from build123d import *

# Parameters (mm, degrees)
BOSS_EXTRUDE1_DEPTH = 104.85
CUT_EXTRUDE1_REACH  = 178.992
CUT_EXTRUDE2_REACH  = 178.992
SKETCH3_R           = 2.665000000000001
BOSS_EXTRUDE2_DEPTH = 104.85
CUT_EXTRUDE3_REACH  = 178.992
SKETCH6_W           = 66.67499999999998
SKETCH6_H           = 36.500000000000014
CUT_EXTRUDE4_DEPTH  = 3.5
CUT_EXTRUDE5_DEPTH  = 94.850000094
SKETCH9_R           = 2.7500000000000084
SKETCH9_R_2         = 2.750000000000008
CUT_EXTRUDE6_DEPTH  = 5
CUT_EXTRUDE7_DEPTH  = 99.85
BOSS_EXTRUDE3_DEPTH = 40
SKETCH12_R          = 19.05
BOSS_EXTRUDE4_DEPTH = 76.2
CHAMFER1_SIZE       = 13.43611593
CHAMFER1_SIZE_2     = 76.2
CUT_EXTRUDE8_REACH  = 166.091
SKETCH13_R          = 8.750000000000004
CUT_EXTRUDE9_REACH  = 166.091
SKETCH14_R          = 1.7500000000000038
SKETCH14_R_2        = 1.7500000000000067
SKETCH14_R_3        = 1.7499999999999987


# Read off the part's stored shape, not the designer's step: Shell1
with BuildPart() as part:
    # Sketch1 → Boss-Extrude1 (new body)
    with BuildSketch(Plane.XY):
        with BuildLine():
            Line((-34.925, 0), (-34.92499999999999, -63.5))
            Line((-34.92499999999999, -63.5), (-34.92499999999998, -103.175))
            Line((-34.92499999999998, -103.175), (98.425, -103.175))
            Line((98.425, -103.175), (98.42499999999998, -64.83388883768319))
            Line((98.42499999999998, -64.83388883768319), (98.425, 0))
            ThreePointArc((98.425, 0), (31.750000000000004, 66.675), (-34.925, 0))
        make_face()
    extrude(amount=BOSS_EXTRUDE1_DEPTH)

    # Sketch2 → Cut-Extrude1 (cut, up to next)
    with BuildSketch(Plane.XY.offset(104.85), mode=Mode.PRIVATE) as cut_extrude1_sk1:
        with BuildLine():
            Line((31.75, -66.675), (31.75, -103.175))
            Line((31.75, -103.175), (98.425, -103.175))
            Line((98.425, -103.175), (98.425, 0))
            ThreePointArc((98.425, 0), (78.89634463561305, -47.14634463561305), (31.75, -66.675))
        make_face()
    cut_extrude1_tool1 = extrude(cut_extrude1_sk1.sketch, amount=-CUT_EXTRUDE1_REACH, mode=Mode.PRIVATE) & part.part
    add(cut_extrude1_tool1.solids().sort_by_distance((70.281775, -75.59134, 104.85))[0], mode=Mode.SUBTRACT)

    # Sketch3 → Cut-Extrude2 (cut, up to next)
    with BuildSketch(Plane(origin=(0, 0, 0), x_dir=(-1, 0, 0), z_dir=(0, 0, -1)), mode=Mode.PRIVATE) as cut_extrude2_sk1:
        with Locations((-21.75, -93.17500000000001)):
            Circle(SKETCH3_R)
    cut_extrude2_tool1 = extrude(cut_extrude2_sk1.sketch, amount=-CUT_EXTRUDE2_REACH, mode=Mode.PRIVATE) & part.part
    # Sketch3 → Cut-Extrude2 (cut, up to next)
    with BuildSketch(Plane(origin=(0, 0, 0), x_dir=(-1, 0, 0), z_dir=(0, 0, -1)), mode=Mode.PRIVATE) as cut_extrude2_sk2:
        with Locations(Location((-21.75, -73.17499999999998, 0), (0, 0, 180))):
            Circle(SKETCH3_R)
    cut_extrude2_tool2 = extrude(cut_extrude2_sk2.sketch, amount=-CUT_EXTRUDE2_REACH, mode=Mode.PRIVATE) & part.part
    # Sketch3 → Cut-Extrude2 (cut, up to next)
    with BuildSketch(Plane(origin=(0, 0, 0), x_dir=(-1, 0, 0), z_dir=(0, 0, -1)), mode=Mode.PRIVATE) as cut_extrude2_sk3:
        with Locations(Location((24.924999999999997, -93.17500000000001, 0), (0, 0, 180))):
            Circle(SKETCH3_R)
    cut_extrude2_tool3 = extrude(cut_extrude2_sk3.sketch, amount=-CUT_EXTRUDE2_REACH, mode=Mode.PRIVATE) & part.part
    # Sketch3 → Cut-Extrude2 (cut, up to next)
    with BuildSketch(Plane(origin=(0, 0, 0), x_dir=(-1, 0, 0), z_dir=(0, 0, -1)), mode=Mode.PRIVATE) as cut_extrude2_sk4:
        with Locations((24.924999999999997, -73.17499999999998)):
            Circle(SKETCH3_R)
    cut_extrude2_tool4 = extrude(cut_extrude2_sk4.sketch, amount=-CUT_EXTRUDE2_REACH, mode=Mode.PRIVATE) & part.part
    add(cut_extrude2_tool1.solids().sort_by_distance((21.75, -93.175, 0))[0], mode=Mode.SUBTRACT)
    add(cut_extrude2_tool2.solids().sort_by_distance((21.75, -73.175, 0))[0], mode=Mode.SUBTRACT)
    add(cut_extrude2_tool3.solids().sort_by_distance((-24.925, -93.175, 0))[0], mode=Mode.SUBTRACT)
    add(cut_extrude2_tool4.solids().sort_by_distance((-24.925, -73.175, 0))[0], mode=Mode.SUBTRACT)

    # Sketch5 → Boss-Extrude2 (add)
    with BuildSketch(Plane(origin=(0, 0, 0), x_dir=(-1, 0, 0), z_dir=(0, 0, -1))):
        with BuildLine():
            Line((-31.75, -66.675), (-98.425, -66.675))
            Line((-98.425, -66.675), (-98.425, -4.6559e-13))
            ThreePointArc((-98.425, -4.6559e-13), (-78.89634463561288, -47.146344635613225), (-31.75, -66.675))
        make_face()
    extrude(amount=-BOSS_EXTRUDE2_DEPTH)

    # Sketch6 → Cut-Extrude3 (cut, up to next)
    with BuildSketch(Plane(origin=(0, 0, 0), x_dir=(-1, 0, 0), z_dir=(0, 0, -1)), mode=Mode.PRIVATE) as cut_extrude3_sk1:
        with Locations((1.5874999999999897, -84.92500000000001)):
            Rectangle(SKETCH6_W, SKETCH6_H)
    cut_extrude3_tool1 = extrude(cut_extrude3_sk1.sketch, amount=-CUT_EXTRUDE3_REACH, mode=Mode.PRIVATE) & part.part
    add(cut_extrude3_tool1.solids().sort_by_distance((-1.5875, -84.925, 0))[0], mode=Mode.SUBTRACT)

    # Sketch7 → Cut-Extrude4 (cut)
    with BuildSketch(Plane.XZ.offset(66.675)):
        Polygon((98.425, 0), (98.425, 104.85), (-34.92499999999999, 104.85), (-34.92499999999998, 0), align=None)
    extrude(amount=-CUT_EXTRUDE4_DEPTH, mode=Mode.SUBTRACT)

    # Sketch8 → Cut-Extrude5 (cut)
    with BuildSketch(Plane(origin=(0, 0, 4.999999905999999), x_dir=(-1, 0, 0), z_dir=(0, 0, -1))):
        with BuildLine():
            Line((-98.425, -20.224984548819855), (-98.425, -60.17499999999999))
            Line((-98.425, -60.17499999999999), (-66.87228637204589, -60.17499999999999))
            ThreePointArc((-66.87228637204589, -60.17500000000001), (-86.42790057980886, -43.18486787272293), (-98.42499999999998, -20.224984548819855))
        make_face()
    extrude(amount=-CUT_EXTRUDE5_DEPTH, mode=Mode.SUBTRACT)

    # Sketch9 → Cut-Extrude6 (cut)
    with BuildSketch(Plane(origin=(0, -60.17499999999999, 0), x_dir=(1, 0, 0), z_dir=(0, 1, 0))):
        with Locations(Location((89.99999999999999, -89.85, 0), (0, 0, 270))):
            Circle(SKETCH9_R)
        with Locations(Location((89.99999999999999, -14.999999906000001, 0), (0, 0, 270))):
            Circle(SKETCH9_R_2)
        with Locations(Location((89.99999999999999, -52.42499995300001, 0), (0, 0, 270))):
            Circle(SKETCH9_R)
    extrude(amount=-CUT_EXTRUDE6_DEPTH, mode=Mode.SUBTRACT)

    # Sketch10 → Cut-Extrude7 (cut)
    with BuildSketch(Plane.XY.offset(104.85)):
        with BuildLine():
            Line((58.2823809623914, -63.175), (80.527879915601, -40.92950104679029))
            ThreePointArc((80.527879915601, -40.92950104679029), (91.58492762854266, -21.778132626262114), (95.425, -4.6274e-13))
            ThreePointArc((95.42499999999998, -4.6803e-13), (31.75000000000024, 63.67499999999998), (-31.92499999999999, 1.274e-14))
            Line((-31.924999999999994, 7.8e-15), (-31.924999999999994, -63.175))
            Line((-31.924999999999994, -63.175), (31.750000000000004, -63.175))
            Line((31.75, -63.175), (58.2823809623914, -63.175))
        make_face()
    extrude(amount=-CUT_EXTRUDE7_DEPTH, mode=Mode.SUBTRACT)

    # Sketch11 → Boss-Extrude3 (add)
    with BuildSketch(Plane.XZ.offset(63.175)):
        Polygon((-34.92499999999999, 104.85), (-31.924999999999994, 104.85), (-31.924999999999994, 20.5), (-34.92499999999998, 20.5), align=None)
    extrude(amount=BOSS_EXTRUDE3_DEPTH)

    # Sketch12 → Boss-Extrude4 (add)
    with BuildSketch(Plane.XY.offset(5)):
        with Locations(Location((31.75, 0, 0), (0, 0, 180))):
            Circle(SKETCH12_R)
    extrude(amount=BOSS_EXTRUDE4_DEPTH)

    # Chamfer1
    # the kernel refuses this chamfer: 76.2, 13.43611593 mm, written as the material it adds along each edge
    with BuildSketch(Plane(origin=(31.75, 0, 5), x_dir=(-1, 1.2e-16, 0), z_dir=(1.2e-16, 1, 0))) as chamfer1_piece_1_section:
        Polygon((19.05 + CHAMFER1_SIZE, 0), (19.05, CHAMFER1_SIZE_2), (19.05, 0), align=None)
    chamfer1_piece_1 = revolve(axis=Axis((31.75, 0, 5), (0, 0, 1)), mode=Mode.PRIVATE)
    chamfer1_piece_1 = split(chamfer1_piece_1, bisect_by=Plane(origin=(57.33414853673409, -6.27e-15, 81.2), z_dir=(0, 0, -1)), keep=Keep.TOP, mode=Mode.PRIVATE)
    add(chamfer1_piece_1)

    # Shell1 outline → Shell1 (revolve, cut)
    with BuildSketch(Plane(origin=(31.75, 0, 0), x_dir=(1, 0, 0), z_dir=(0, -1, 0))):
        Polygon((14.854501844, 76.2), (0, 76.2), (0, 0), (28.290617774, 0), align=None)
    revolve(axis=Axis((31.75, 0, 0), (0, 0, 1)), mode=Mode.SUBTRACT)

    # Sketch13 → Cut-Extrude8 (cut, up to next)
    with BuildSketch(Plane.XY.offset(81.2), mode=Mode.PRIVATE) as cut_extrude8_sk1:
        with Locations((31.75, 0)):
            Circle(SKETCH13_R)
    cut_extrude8_tool1 = extrude(cut_extrude8_sk1.sketch, amount=-CUT_EXTRUDE8_REACH, mode=Mode.PRIVATE) & part.part
    add(cut_extrude8_tool1.solids().sort_by_distance((31.75, 0, 81.2))[0], mode=Mode.SUBTRACT)

    # Sketch14 → Cut-Extrude9 (cut, up to next)
    with BuildSketch(Plane.XY.offset(81.2), mode=Mode.PRIVATE) as cut_extrude9_sk1:
        with Locations((31.75, 10.999999999999993)):
            Circle(SKETCH14_R)
    cut_extrude9_tool1 = extrude(cut_extrude9_sk1.sketch, amount=-CUT_EXTRUDE9_REACH, mode=Mode.PRIVATE) & part.part
    # Sketch14 → Cut-Extrude9 (cut, up to next)
    with BuildSketch(Plane.XY.offset(81.2), mode=Mode.PRIVATE) as cut_extrude9_sk2:
        with Locations((42.75000000000015, 1.1102e-13)):
            Circle(SKETCH14_R)
    cut_extrude9_tool2 = extrude(cut_extrude9_sk2.sketch, amount=-CUT_EXTRUDE9_REACH, mode=Mode.PRIVATE) & part.part
    # Sketch14 → Cut-Extrude9 (cut, up to next)
    with BuildSketch(Plane.XY.offset(81.2), mode=Mode.PRIVATE) as cut_extrude9_sk3:
        with Locations((31.75000000000024, -10.999999999999993)):
            Circle(SKETCH14_R_2)
    cut_extrude9_tool3 = extrude(cut_extrude9_sk3.sketch, amount=-CUT_EXTRUDE9_REACH, mode=Mode.PRIVATE) & part.part
    # Sketch14 → Cut-Extrude9 (cut, up to next)
    with BuildSketch(Plane.XY.offset(81.2), mode=Mode.PRIVATE) as cut_extrude9_sk4:
        with Locations((20.75000000000016, -3.469e-14)):
            Circle(SKETCH14_R_3)
    cut_extrude9_tool4 = extrude(cut_extrude9_sk4.sketch, amount=-CUT_EXTRUDE9_REACH, mode=Mode.PRIVATE) & part.part
    add(cut_extrude9_tool1.solids().sort_by_distance((31.75, 11, 81.2))[0], mode=Mode.SUBTRACT)
    add(cut_extrude9_tool2.solids().sort_by_distance((42.75, 0, 81.2))[0], mode=Mode.SUBTRACT)
    add(cut_extrude9_tool3.solids().sort_by_distance((31.75, -11, 81.2))[0], mode=Mode.SUBTRACT)
    add(cut_extrude9_tool4.solids().sort_by_distance((20.75, 0, 81.2))[0], mode=Mode.SUBTRACT)


solid = part.part
Geometry: final body of the model. Coordinates: model frame, mm. A direction names the side the tool comes from. Coordinates: 2 decimals unless noted, no trailing zeros. Order: outer loops, then holes, each group sorted by start corner. A loop starts at its lowest first (then second) coordinate and runs counter-clockwise, first axis right, second up.
1) Section C-C (x = 71). Return loops of the section in (y, z) (3 decimals).
Result sheet:
outline: (-63.175, 0) - (53.898, 0) - (53.898, 104.85) - (50.139, 104.85) - (50.139, 5) - (-50.457, 5) - (-50.457, 104.85) - (-63.175, 104.85) - close; hole (-60.175, 5) - (-57.568, 5) - (-57.568, 99.85) - (-60.175, 99.85) - close
2) Draft query along Z for faces 1 (the cylindrical face through (87.56, -61.65, 53.69)), 2 (the flat face through (46, -26, 0)), 3 (the flat face through (27.8, 8.2, 81.2)), 4 (the cylindrical face through (40.096, 2.628, 78.735)). Return one class per face: released by +Z, released by -Z, zero draft, split by the parting line, or undercut.
Result sheet:
face 1: undercut
face 2: released by -Z
face 3: released by +Z
face 4: zero draft
3) Section B-B (x = 90). Return loops of the section in (y, z) (3 decimals), then the cut area to 3 significant figures.
Result sheet:
outline: (-63.175, 0) - (32.442, 0) - (32.442, 104.85) - (25.719, 104.85) - (25.719, 5) - (-25.719, 5) - (-25.719, 104.85) - (-63.175, 104.85) - (-63.175, 92.6) - (-60.175, 92.6) - (-60.175, 99.85) - (-38.23, 99.85) - (-38.23, 5) - (-60.175, 5) - (-60.175, 12.25) - (-63.175, 12.25) - close; (-63.175, 17.75) - (-60.175, 17.75) - (-60.175, 49.675) - (-63.175, 49.675) - close; (-63.175, 55.175) - (-60.175, 55.175) - (-60.175, 87.1) - (-63.175, 87.1) - close
area: 2,760 mm2
4) Section A-A (z = 9). Give the number of separate pieces and of enclosed holes in the cut face, then the cut area to 3 significant figures.
Result sheet:
separate pieces: 2
enclosed holes: 1
area: 2,230 mm2
5) Ray query, probe 1 along Z at (x, y) = (90, -61.3) (3 decimals); probe 2 along Y at (x, z) = (16.5, 56.5); probe 3 along X at (y, z) = (20.5, 15.5). Return the intervals inside material, ascending.
Result sheet:
probe 1: z = 0 to 12.25, 17.75 to 49.675, 55.175 to 87.1, 92.6 to 104.85
probe 2: y = -17.76 to -10.17, 10.17 to 17.76, 61.82 to 64.91
probe 3: x = -31.7 to -28.53, 8.99 to 16.49, 47.01 to 54.51, 92.03 to 95.2
6) Set-up query: faces 5 (the flat face through (-31.925, -51, 56)), 6 (the flat face through (2.6, 15.2, 5)), 7 (the cylindrical face through (87.315, -61.654, 14.404)), 8 (the flat face through (90, -49, 99.85)), 9 (the flat face through (38.1, -6.4, 76.2)). Return all of +Z, -Z, +X, -X, +Y, -Y with unobstructed straight access to the full face (end or side cutting, diameter ignored); none if empty.
Result sheet:
face 5: +Z, -Y
face 6: +Z
face 7: -Y
face 8: +X
face 9: -Z
7) First-contact query: P1, Ø2.5, axis at x = -33, y = -75, coming from the -Z side; P2, Ø1.5, axis at x = 40, y = 49, coming from the +Z side; P3, Ø1.5, axis at y = 23, z = 33, coming from the -X side; P4, Ø5, axis at x = 8.5, y = -55, coming from the -Z side. Flat tips, straight axial feed; report the tip coordinate or a pass-through.
Result sheet:
P1: stops at z = 20.5
P2: stops at z = 5
P3: stops at x = -31.1
P4: stops at z = 0
